Part model, mm, in its own coordinate system. A direction names the side the tool comes from. Round coordinates to 2 decimals unless told otherwise and drop trailing zeros. Order: outer loops, then holes, each group sorted by start corner. A loop starts at its lowest first (then second) coordinate and runs counter-clockwise, first axis right, second up. Notation, with made-up numbers: (88.5, 87.25) - (120.5, 87.25) arc R22 ccw to (120.5, 114.25) - close; hole circle Ø3 at (19, 28). An arc over 180 degrees is marked (long way). Answer as a JSON object with one key per item and string values.
```python
from build123d import *

# Parameters (mm, degrees)
F0_W         = 90
F0_H         = 77
F1_DEPTH     = 22
F0_W_2       = 100
F0_H_2       = 87
F2_DEPTH     = 42
F3_R         = 14
F4_R         = 5
F5_R         = 5
F6_T1_DEPTH  = 72
F6_T3_DEPTH  = 59
F6_T6_ANGLE  = 90
F6_T8_ANGLE  = 90
F6_T10_ANGLE = 90
F6_T12_ANGLE = 90


# Not quite as in the source:
# - a fillet or chamfer that OpenCascade refuses, or shapes differently, is made with other operations: its cross-section is extruded or revolved along the edge and cut away or added


with BuildPart() as f1:
    # F0 (on Top) → F1 (new body)
    with BuildSketch(Plane.XY):
        Rectangle(F0_W, F0_H)
    extrude(amount=F1_DEPTH)

    # F0 (on Top) → F2 (join)
    with BuildSketch(Plane.XY):
        Rectangle(F0_W_2, F0_H_2)
        Rectangle(F0_W, F0_H, mode=Mode.SUBTRACT)
    extrude(amount=F2_DEPTH)

    # F3
    f3_edges = [f1.edges().sort_by_distance(p)[0] for p in [
        (-50, -43.5, 21),
        (-50, 43.5, 21),
        (50, 43.5, 21),
        (50, -43.5, 21),
    ]]
    fillet(f3_edges, radius=F3_R)

    # F4
    f4_edges = [f1.edges().sort_by_distance(p)[0] for p in [
        (0, 43.5, 0),
    ]]
    fillet(f4_edges, radius=F4_R)

    # F5
    f5_edges = [f1.edges().sort_by_distance(p)[0] for p in [
        (-45, -38.5, 32),
        (45, -38.5, 32),
        (-45, 38.5, 32),
        (45, 38.5, 32),
    ]]
    fillet(f5_edges, radius=F5_R)

    # F6: fillet of radius 5 on 8 edges, made by hand

    # F6_s2 → F6_t1 (cut)
    with BuildSketch(Plane.YZ.offset(-36)):
        with BuildLine():
            ThreePointArc((-38.5, 42), (-42.0355339059, 40.5355339059), (-43.5, 37))
            Line((-43.5, 37), (-43.5, 42))
            Line((-43.5, 42), (-38.5, 42))
        make_face()
        with BuildLine():
            ThreePointArc((38.5, 42), (42.0355339059, 40.5355339059), (43.5, 37))
            Line((43.5, 37), (43.5, 42))
            Line((43.5, 42), (38.5, 42))
        make_face()
    extrude(amount=F6_T1_DEPTH, mode=Mode.SUBTRACT)

    # F6_s4 → F6_t3 (cut)
    with BuildSketch(Plane.XZ.offset(-29.5)):
        with BuildLine():
            ThreePointArc((45, 42), (48.5355339059, 40.5355339059), (50, 37))
            Line((50, 37), (50, 42))
            Line((50, 42), (45, 42))
        make_face()
        with BuildLine():
            ThreePointArc((-45, 42), (-48.5355339059, 40.5355339059), (-50, 37))
            Line((-50, 37), (-50, 42))
            Line((-50, 42), (-45, 42))
        make_face()
    extrude(amount=F6_T3_DEPTH, mode=Mode.SUBTRACT)

    # F6_s5 → F6_t6 (revolve, cut)
    with BuildSketch(Plane.XZ.offset(29.5)):
        with BuildLine():
            ThreePointArc((45, 42), (48.5355339059, 40.5355339059), (50, 37))
            Line((50, 37), (50, 42))
            Line((50, 42), (45, 42))
        make_face()
    revolve(axis=Axis((36, -29.5, 42), (0, 0, -1)), revolution_arc=F6_T6_ANGLE, mode=Mode.SUBTRACT)

    # F6_s7 → F6_t8 (revolve, cut)
    with BuildSketch(Plane.XZ.offset(-29.5)):
        with BuildLine():
            ThreePointArc((45, 42), (48.5355339059, 40.5355339059), (50, 37))
            Line((50, 37), (50, 42))
            Line((50, 42), (45, 42))
        make_face()
    revolve(axis=Axis((36, 29.5, 42), (0, 0, 1)), revolution_arc=F6_T8_ANGLE, mode=Mode.SUBTRACT)

    # F6_s9 → F6_t10 (revolve, cut)
    with BuildSketch(Plane.XZ.offset(29.5)):
        with BuildLine():
            ThreePointArc((-45, 42), (-48.5355339059, 40.5355339059), (-50, 37))
            Line((-50, 37), (-50, 42))
            Line((-50, 42), (-45, 42))
        make_face()
    revolve(axis=Axis((-36, -29.5, 42), (0, 0, 1)), revolution_arc=F6_T10_ANGLE, mode=Mode.SUBTRACT)

    # F6_s11 → F6_t12 (revolve, cut)
    with BuildSketch(Plane.YZ.offset(-36)):
        with BuildLine():
            ThreePointArc((38.5, 42), (42.0355339059, 40.5355339059), (43.5, 37))
            Line((43.5, 37), (43.5, 42))
            Line((43.5, 42), (38.5, 42))
        make_face()
    revolve(axis=Axis((-36, 29.5, 42), (0, 0, 1)), revolution_arc=F6_T12_ANGLE, mode=Mode.SUBTRACT)


solid = f1.part
```
Item 1: Cut at D-D (z = 29.5). Write the cut outline in (x, y).
Taken from the geometry:
{"outline": "(-50, -29.5) arc R14 ccw to (-36, -43.5) - (36, -43.5) arc R14 ccw to (50, -29.5) - (50, 29.5) arc R14 ccw to (36, 43.5) - (-36, 43.5) arc R14 ccw to (-50, 29.5) - close; hole (-45, -33.5) arc R5 ccw to (-40, -38.5) - (40, -38.5) arc R5 ccw to (45, -33.5) - (45, 33.5) arc R5 ccw to (40, 38.5) - (-40, 38.5) arc R5 ccw to (-45, 33.5) - close"}
Item 2: Cut at C-C (x = 34). Write the cut outline in (y, z).
Taken from the geometry:
{"outline": "(-43.5, 5) arc R5 ccw to (-38.5, 0) - (38.5, 0) arc R5 ccw to (43.5, 5) - (43.5, 37) arc R5 ccw to (38.5, 42) - (38.5, 22) - (-38.5, 22) - (-38.5, 42) arc R5 ccw to (-43.5, 37) - close"}
Item 3: Drop flat-ended pins along their axis: P1, Ø1, axis at y = 32, z = 7, coming from the -X side; P2, Ø23, axis at x = 0, y = -15, coming from the +Z side; P3, Ø8, axis at y = -33.5, z = 8, coming from the +X side. Give the stop position or say it passes through.
Taken from the geometry:
{"P1": "x = -49.86", "P2": "z = 22", "P3": "x = 50"}
Item 4: Two-plate mould, pull along X, no slides. Class faces 3 (the flat face through (-1, -38.5, 32)), 4 (the cylindrical face through (-0.5, -42, 40.57)), 5 (the flat face through (50, 0, 21)): pulls with the +X half, pulls with the -X half, needs draft (parallel to the pull), parting line crosses it, or undercut.
Taken from the geometry:
{"face 3": "undercut", "face 4": "needs draft", "face 5": "pulls with the +X half"}
Item 5: Tool access for faces 1 (the flat face through (45, 0, 32)), 2 (the flat face through (-1, -43.5, 21)): list every direction of +Z, -Z, +X, -X, +Y, -Y with a clear straight run to the whole face (end or side of a thin tool).
Taken from the geometry:
{"face 1": "+Z", "face 2": "+Z, -Z, +X, -X, -Y"}
Item 6: Cut at A-A (y = -7). Write the cut outline in (x, z).
Taken from the geometry:
{"outline": "(-50, 5) arc R5 ccw to (-45, 0) - (45, 0) arc R5 ccw to (50, 5) - (50, 37) arc R5 ccw to (45, 42) - (45, 22) - (-45, 22) - (-45, 42) arc R5 ccw to (-50, 37) - close"}
Item 7: Cut at B-B (z = 9.5). Write the cut outline in (x, y), plus the area to 3 significant figures.
Taken from the geometry:
{"outline": "(-50, -29.5) arc R14 ccw to (-36, -43.5) - (36, -43.5) arc R14 ccw to (50, -29.5) - (50, 29.5) arc R14 ccw to (36, 43.5) - (-36, 43.5) arc R14 ccw to (-50, 29.5) - close", "area": "8,530 mm2"}
Item 8: Probe L1, parallel to Y at x = -16.5, z = 37; L2, parallel to X at y = 29, z = 27.5; L3, parallel to Z at x = -9.5, y = -39. List the from-to ranges inside material, lowest first. Write a range as from..to.
Taken from the geometry:
{"L1": "-43.5..-38.5, 38.5..43.5", "L2": "-50..-45, 45..50", "L3": "0.03..41.97"}
